```python
from build123d import *

# Parameters (mm, degrees)
SKETCH1_W           = 20
SKETCH1_H           = 20
BOSS_EXTRUDE1_DEPTH = 10


with BuildPart() as part:
    # Sketch1 → Boss-Extrude1 (new body)
    with BuildSketch(Plane(origin=(0, 0, 0), x_dir=(1, 0, 0), z_dir=(0, 1, 0))):
        with BuildLine():
            Line((23.939871077, 2.849965846), (42.576368333, -0.125028462))
            ThreePointArc((42.576368333, -0.125028462), (51, -10), (42.576368333, -19.874971538))
            Line((42.576368333, -19.874971538), (30.394725659, -21.819560004))
            ThreePointArc((30.394725659, -21.819560004), (24.408108439, -24.617839175), (20.810680125, -30.161165034))
            Line((20.810680125, -30.161165034), (15.737843767, -46.754180408))
            ThreePointArc((15.737843767, -46.754180408), (10, -51), (4.262156233, -46.754180408))
            Line((4.262156233, -46.754180408), (-2.475687534, -24.71500206))
            ThreePointArc((-2.475687534, -24.71500206), (-2.868198061, -22.980302653), (-3, -21.206641244))
            Line((-3, -21.206641244), (-3, 1))
            ThreePointArc((-3, 1), (-2.414213562, 2.414213562), (-1, 3))
            Line((-1, 3), (22.048229077, 3))
            ThreePointArc((22.048229077, 3), (22.997020375, 2.962432657), (23.939871077, 2.849965846))
        make_face()
        with Locations((10, -10)):
            Rectangle(SKETCH1_W, SKETCH1_H, mode=Mode.SUBTRACT)
    extrude(amount=BOSS_EXTRUDE1_DEPTH)


solid = part.part
```
CAD build for the part. Positions are in the model's coordinates, mm. A direction names the side the tool comes from. Round coordinates to 2 decimals unless told otherwise and drop trailing zeros. Loops run counter-clockwise (first coordinate to the right, second up) from the corner with the lowest first, then second, coordinate; pieces in that order, holes last. Notation, with made-up numbers: M 24.5,12 L 82.5,12 A23 cw 82.5,51 Z; hole C -24.75,80.5 d11. An arc over 180 degrees is marked long. Use a Markdown table: item, result. Add a question column.
(1) Pull direction X, two halves, no side cores. Call faces 1 (the face through (10, 5, 51)), 2 (the face through (36.571, 4.93, 20.834)), 3 (the face through (0, 5, 10)), 4 (the face through (20, 5, 10)): +X half, -X half, draft (parallel to the pull), parting line (faces both ways), or undercut.
(2) Cut at C-C (x = 8). Give the cut face in (y, z), and give its area (3 significant figures).
(3) Flat gauge pins, fed straight in: pin 1 (5 mm diameter, centred on y = 2, z = 36, fed in from -X); pin 2 (4 mm diameter, centred on y = 7, z = 33.5, fed in from +X); pin 3 (8 mm diameter, centred on x = 9, z = 4.5, fed in from +Y); pin 4 (3 mm diameter, centred on y = 6.5, z = 5.5, fed in from +X). Where does each tip first touch, or does it go through?
(4) Drill centre lines: line 1 (X direction, y = 7.75, z = 10.5); line 2 (Z direction, x = 12, y = 5.25); line 3 (Z direction, x = 5.5, y = 8.5). Where is each one in solid material? Low to high.
(5) Cut at A-A (y = 2.75). Give the cut face in (x, z) (3 decimals), and give its area (3 significant figures).
(6) Which spindle directions (+Z, -Z, +X, -X, +Y, -Y) get a long thin tool onto all of the face, cutting with end or side? Do faces 5 (the face through (10, 5, -3)), 6 (the face through (10, 5, 0)). Say none if no direction does.
(7) Cut at B-B (x = 13.5). Give the cut face in (y, z), and give its area (3 significant figures).
(8) Cut at D-D (z = 34.5). Give the cut face in (x, y).
Geometry says:
| question | item | result |
|---|---|---|
| 1 | face 1 | parting line |
| 1 | face 2 | +X half |
| 1 | face 3 | undercut |
| 1 | face 4 | undercut |
| 2 | outline | M 0,-3 L 10,-3 L 10,0 L 0,0 Z; M 0,20 L 10,20 L 10,50.66 L 0,50.66 Z |
| 2 | area | 337 mm² |
| 3 | pin 1 | stops at x = 0.21 |
| 3 | pin 2 | stops at x = 20.4 |
| 3 | pin 3 | passes through |
| 3 | pin 4 | stops at x = 50.54 |
| 4 | line 1 | x = -3 to 0, 20 to 50.99 |
| 4 | line 2 | z = -3 to 0, 20 to 50.66 |
| 4 | line 3 | z = -3 to 0, 20 to 48.97 |
| 5 | outline | M -3,-1 A2 ccw -1,-3 L 22.048,-3 A12 ccw 23.94,-2.85 L 42.576,0.125 A10 ccw 42.576,19.875 L 30.395,21.82 A12 cw 20.811,30.161 L 15.738,46.754 A6 ccw 4.262,46.754 L -2.476,24.715 A12 ccw -3,21.207 Z; hole M 0,0 L 20,0 L 20,20 L 0,20 Z |
| 5 | area | 1,340 mm² |
| 6 | face 5 | -Z, +X, -X, +Y, -Y |
| 6 | face 6 | +Y, -Y |
| 7 | outline | M 0,-3 L 10,-3 L 10,0 L 0,0 Z; M 0,20 L 10,20 L 10,49.87 L 0,49.87 Z |
| 7 | area | 329 mm² |
| 8 | outline | M 0.52,0 L 19.48,0 L 19.48,10 L 0.52,10 Z |
